```python
from build123d import *

# Parameters (mm, degrees)
PAD_DEPTH       = 90
POCKET_DEPTH    = 45
SKETCH002_W     = 40
SKETCH002_H     = 57
POCKET001_DEPTH = 45
SKETCH003_R     = 10.5
SKETCH003_W     = 18
SKETCH003_H     = 8
POCKET002_DEPTH = 40
FILLET_R        = 6
FILLET001_R     = 3
FILLET002_R     = 4
FILLET003_R     = 3
FILLET004_R     = 3


with BuildPart() as part:
    # Sketch → Pad (new body, symmetric)
    with BuildSketch(Plane.XY):
        Polygon((-55, 50), (0, 65), (0, -65), (-55, -50), align=None)
    extrude(amount=PAD_DEPTH, both=True)

    # Sketch001 (on Face4 of Pad) → Pocket (cut)
    with BuildSketch(Plane(origin=(-55, 0, 0), x_dir=(0, -1, 0), z_dir=(-1, 0, 0))):
        Polygon((7.870361, 81.046063), (27.870361, 81.046063), (27.706422, -63.953844), (7.870361, -63.953844), align=None)
    extrude(amount=-POCKET_DEPTH, mode=Mode.SUBTRACT)

    # Sketch002 (on Face2 of Pocket) → Pocket001 (cut)
    with BuildSketch(Plane(origin=(-55, 0, 0), x_dir=(0, -1, 0), z_dir=(-1, 0, 0))):
        with Locations((-24.249742, 42.474102)):
            Rectangle(SKETCH002_W, SKETCH002_H)
    extrude(amount=-POCKET001_DEPTH, mode=Mode.SUBTRACT)

    # Sketch003 (on Face2 of Pocket001) → Pocket002 (cut)
    with BuildSketch(Plane(origin=(-55, 0, 0), x_dir=(0, -1, 0), z_dir=(-1, 0, 0))):
        with Locations((-24.992333, -20.97492)):
            Circle(SKETCH003_R)
        with Locations((-24.674738, -49.574854)):
            Circle(SKETCH003_R)
        with Locations((-26.581285, -76.962609)):
            Rectangle(SKETCH003_W, SKETCH003_H)
    extrude(amount=-POCKET002_DEPTH, mode=Mode.SUBTRACT)

    # Fillet
    fillet_edges = [part.edges().sort_by_distance(p)[0] for p in [
        (-27.5, -57.5, -90),
        (-27.5, 57.5, -90),
        (-55, 50, 0),
        (-55, -50, 0),
        (-55, 0, -90),
        (-55, 0, 90),
        (-27.5, -57.5, 90),
        (-27.5, 57.5, 90),
    ]]
    fillet(fillet_edges, radius=FILLET_R)

    # Fillet001
    fillet001_edges = [part.edges().sort_by_distance(p)[0] for p in [
        (-55, 35.492333, -20.97492),
        (-55, 35.174738, -49.574854),
    ]]
    fillet(fillet001_edges, radius=FILLET001_R)

    # Fillet002
    fillet002_edges = [part.edges().sort_by_distance(p)[0] for p in [
        (-55, -27.788392, 8.546109),
        (-55, -7.870361, 8.546109),
    ]]
    fillet(fillet002_edges, radius=FILLET002_R)

    # Fillet003
    fillet003_edges = [part.edges().sort_by_distance(p)[0] for p in [
        (-55, 4.249742, 42.474102),
        (-55, 24.249742, 70.974102),
        (-55, 24.249742, 13.974102),
    ]]
    fillet(fillet003_edges, radius=FILLET003_R)

    # Fillet004
    fillet004_edges = [part.edges().sort_by_distance(p)[0] for p in [
        (-55, 26.581285, -72.962609),
        (-55, 35.581285, -76.962609),
        (-55, 17.581285, -76.962609),
        (-55, 26.581285, -80.962609),
    ]]
    fillet(fillet004_edges, radius=FILLET004_R)


solid = part.part
```
Read the model definition and answer for the solid it produces. Units are mm, in the model's axes. A direction names the side the tool comes from. Give positions to 0.01 mm unless a question says otherwise; leave off trailing zeros. Write item = value, one per line. Start each with the question number.
Item 1: The mould has two halves that part along Z. Classify faces 3 (the flat face through (-31, 25, 70.974)), 4 (the cylindrical face through (-53.289, 0.636, 88.196)), 5 (the cylindrical face through (-24.485, 56.549, -88.196)): +Z half, -Z half, draft (parallel to the pull), parting line (faces both ways), or undercut.
Item 2: Find the intervals of material crossed by probe 1 along Y at (x, z) = (-18, 21); probe 2 along Y at (x, z) = (-41.5, 39); probe 3 along Z at (x, y) = (-48.5, -18.5), in increasing order. Write a range as [from, to].
Item 3: Find section A-A (x = -24). State how many separate pieces and enclosed holes the cut face has, then the cut area to 3 significant figures.
Item 4: Each of these flat-tipped pins is pushed along its axis until it touches: P1, Ø4, axis at x = -19, z = -25.5, coming from the -Y side; P2, Ø20.5, axis at x = -24, z = 35.5, coming from the -Y side; P3, Ø2, axis at y = 23.5, z = 36.5, coming from the -X side. Where does it stop, or does it pass through?
Item 5: A tool of negligible diameter and unlimited length cuts with its end or side. For faces 1 (the flat face through (-31, 25, 13.974)), 2 (the flat face through (-24, 1, 90)), from which of +Z, -Z, +X, -X, +Y, -Y can it reach the whole face along a straight path? Write none if from no direction.
Response:
q1.face_3 = undercut
q1.face_4 = +Z half
q1.face_5 = -Z half
q2.probe_1 = [-60.09, -27.8], [-7.87, 4.25], [44.25, 60.09]
q2.probe_2 = [-53.68, -27.82], [-7.87, 4.25], [44.25, 53.68]
q2.probe_3 = [-90, -63.95], [81.05, 90]
q3.separate_pieces = 1
q3.enclosed_holes = 5
q3.area = 15,000 mm²
q4.P1 = -60.36
q4.P2 = -61.25
q4.P3 = -10
q5.face_1 = -X
q5.face_2 = +Z, +X, -X, +Y, -Y
